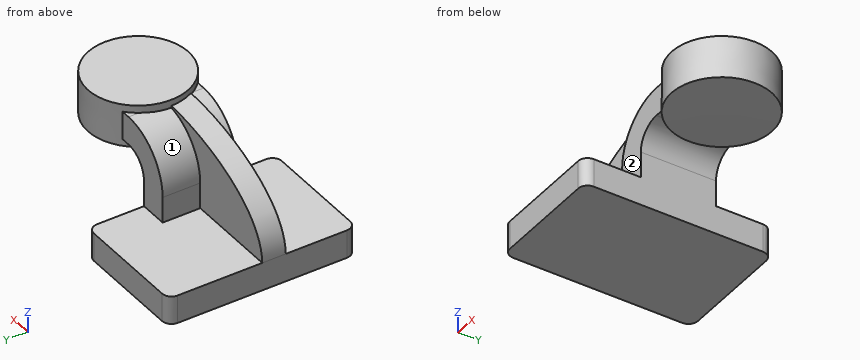
```python
from build123d import *

# Parameters (mm, degrees)
F1_DEPTH = 63.5
F2_DEPTH = 25.4
F3_DEPTH = 15.875
F5_R     = 6.35


with BuildPart() as f1:
    # F0 (on Front) → F1 (new body, symmetric)
    with BuildSketch(Plane.XZ):
        Polygon((22.225, 9.525), (-41.275, 9.525), (-41.275, -9.525), (41.275, -9.525), (41.275, 9.525), align=None)
    extrude(amount=F1_DEPTH, both=True)

    # F0 (on Front) → F2 (join, symmetric)
    with BuildSketch(Plane.XZ):
        with BuildLine():
            Line((22.225, 27.0002), (22.225, 9.525))
            Line((22.225, 9.525), (41.275, 9.525))
            Line((41.275, 9.525), (41.275, 27.0002))
            ThreePointArc((41.275, 27.0002), (45.9246798487, 38.2255201513), (57.15, 42.8752))
            Line((57.15, 42.8752), (68.7600185826, 42.8752))
            Line((68.7600185826, 42.8752), (85.6484008946, 42.8752))
            Line((85.6484008946, 42.8752), (85.7097128786, 61.9252))
            Line((85.7097128786, 61.9252), (68.7600185826, 61.9252))
            Line((68.7600185826, 61.9252), (57.15, 61.9252))
            ThreePointArc((57.15, 61.9252), (32.4542956671, 51.6959043329), (22.225, 27.0002))
        make_face()
    extrude(amount=F2_DEPTH, both=True)

    # F0 (on Front) → F3 (join)
    with BuildSketch(Plane.XZ):
        with BuildLine():
            add(Edge.make_bspline(
                [(-41.275, 9.525), (-39.5817421377, 51.6913831234), (38.1245203316, 67.0281425118), (68.7600185826, 61.9252)],
                knots=[0, 0, 0, 0, 121.8748795877, 121.8748795877, 121.8748795877, 121.8748795877], degree=3))
            Line((-41.275, 9.525), (22.225, 9.525))
            Line((22.225, 9.525), (22.225, 27.0002))
            ThreePointArc((22.225, 27.0002), (32.4542956671, 51.6959043329), (57.15, 61.9252))
            Line((57.15, 61.9252), (68.7600185826, 61.9252))
        make_face()
    extrude(amount=F3_DEPTH)

    # F0 (on Front) → F4 (revolve)
    with BuildSketch(Plane.XZ):
        Polygon((85.725, 66.675), (85.7097128786, 61.9252), (85.6484008946, 42.8752), (85.6330320239, 38.1), (119.5600185826, 38.1), (119.5600185826, 66.675), align=None)
    revolve(axis=Axis((85.679016012, 0, 52.3875), (0.0032184602, 0, 0.9999948207)))

    # F5
    f5_edges = [f1.edges().sort_by_distance(p)[0] for p in [
        (-41.275, -63.5, 0),
        (41.275, -63.5, 0),
        (41.275, 63.5, 0),
        (-41.275, 63.5, 0),
    ]]
    fillet(f5_edges, radius=F5_R)


solid = f1.part
```
The model under review builds one solid part; all positions refer to its coordinate system, in mm. Face numbers are marked on the shaded views. A direction names the side the tool comes from. Round coordinates to 2 decimals unless told otherwise and drop trailing zeros. Loops run counter-clockwise (first coordinate to the right, second up) from the corner with the lowest first, then second, coordinate; pieces in that order, holes last. Notation, with made-up numbers: (-13.75, 9.5) -> (6.25, 9.5) arc R7 cw to (6.25, 13.5) -> close; hole circle Ø7 at (2, 85). An arc over 180 degrees is marked (long way). Answer as a JSON object with one key per item and string values. Group by question number.
1) We need section A-A on y = 41. Write out the cut boundary in (x, z) (3 decimals).
2) For pin 1 Ø1.8 at (x, y) = (60.5, 23) entering from -Z; pin 2 Ø5 at (x, y) = (60.5, 21) entering from +Z; pin 3 Ø20.5 at (x, z) = (40, 48) entering from +Y, all flat-tipped, find the tip position at first contact; note any pin that passes through.
3) For the marked faces 1 and 2, list the 3-axis set-ups (+Z, -Z, +X, -X, +Y, -Y) from which the entire face can be reached by the end or side of a thin tool; tool diameter is ignored.
4) For line 1 (Y direction, x = 35, z = 57.5) (3 decimals); line 2 (Z direction, x = -25, y = 25) (3 decimals); line 3 (X direction, y = 53.5, z = 4) (3 decimals), list the stretches that pass through material, from the lowest coordinate up. Write a range as [from, to].
Result set:
{
 "1": {"outline": "(-41.275, -9.525) -> (41.275, -9.525) -> (41.275, 9.525) -> (-41.275, 9.525) -> close"},
 "2": {"pin 1": "z = 38.29", "pin 2": "z = 66.87", "pin 3": "y = 25.4"},
 "3": {"face 1": "+Z, -X, +Y", "face 2": "+Z, -X, -Y"},
 "4": {"line 1": "[-15.875, 0]", "line 2": "[-9.525, 9.525]", "line 3": "[-41.275, 41.275]"}
}
